Model file for the job. Use its own axes, mm. A direction names the side the tool comes from. Give positions to 0.01 mm unless a question says otherwise; leave off trailing zeros. Use CSV: the item, a comma, the result in double quotes.
Autodesk Inventor part; units mm, degrees
ref_plane "Work Plane1" through (16.3274, 9.3302, 5.6189) normal (-0.0349, 0, -0.9994) x (0, 1, 0)
ref_plane "YZ Plane" through (0, 0, 0) normal (1, 0, 0) x (0, 1, 0)
ref_plane "XZ Plane" through (0, 0, 0) normal (0, 1, 0) x (-1, 0, 0)
sketch "Sketch1" plane through (0, 0, 0) normal (0, 0, 1) x (1, 0, 0)
  line L0 (112.0815, -40.6698) -> (40.0716, -40.6698)
  line L1 (40.0716, -40.6698) -> (40.0716, 86.9433)
  line L2 (40.0716, 86.9433) -> (112.0815, 86.9433)
  line L3 (112.0815, 86.9433) -> (112.0815, -40.6698)
  line L4 (40.0716, -40.6698) -> (50.0716, -40.6698) construction
  point P0 (0, 0)
extrude "Extrusion1" add sketch "Sketch1" along normal blind 5.15
sketch "Sketch2" plane through (0, 0, 5.15) normal (0, 0, 1) x (1, 0, 0)
  point P0 (0, 0)
sketch "Sketch4" plane through (0, 0, 5.15) normal (0, 0, 1) x (1, 0, 0)
  circle A0 centre (102.6515, 97.6673) radius 2.8 construction
  circle A1 centre (53.4593, 78.9433) radius 2.8 construction
  circle A2 centre (55.5115, 50.5273) radius 2.8 construction
  circle A3 centre (102.6515, 50.5273) radius 2.8 construction
  line L0 (53.4593, 78.9433) -> (53.4593, 75.9433) construction
  line L1 (50.6593, 78.9433) -> (50.6593, 75.9433)
  line L2 (56.2593, 75.9433) -> (56.2593, 78.9433)
  arc A4 (56.2593, 78.9433) -> (50.6593, 78.9433) centre (53.4593, 78.9433) ccw
  arc A5 (50.6593, 75.9433) -> (56.2593, 75.9433) centre (53.4593, 75.9433) ccw
  line L3 (40.0716, 86.9433) -> (40.0716, -40.6698)
  line L4 (112.0815, 86.9433) -> (40.0716, 86.9433)
  circle A6 centre (53.4593, 77.3133) radius 5
  line L5 (53.4593, 77.3133) -> (53.4593, 77.5733) construction
  point P0 (0, 0)
  point P1 (53.4593, 77.4433)
  point P2 (40.0716, -42.6698)
  point P3 (53.4593, 77.4433)
  dimension "d7" = 3
  dimension "d27" = 5.6
  dimension "d29" = 8
extrude "Extrusion3" cut sketch "Sketch4" against normal through all contours A4 L2 A5 L1
pattern_linear "Rectangular Pattern1" count 2 spacing 47.14 along (1, 0, 0) count 2 spacing 47.14 along (0, -1, 0) of "Extrusion3"
sketch "Sketch9" plane through (0, 0, 5.15) normal (0, 0, 1) x (1, 0, 0)
  point P0 (55.0716, -3.0051)
  point P1 (44.0716, -3.0051)
  point P2 (44.0716, -19.0051)
  point P3 (44.0716, -35.0051)
  point P4 (44.0716, 36.9949)
hole "Hole1" at (55.0716, -3.0051, 5.15) at (44.0716, -3.0051, 5.15) at (44.0716, -19.0051, 5.15) at (44.0716, -35.0051, 5.15) at (44.0716, 36.9949, 5.15) direction (0, 0, -1) diameter 4.4 depth 5.15
sketch "Sketch12" plane through (0, 0, 5.15) normal (0, 0, 1) x (1, 0, 0)
  line L0 (40.0716, -40.6698) -> (112.0815, -40.6698)
  arc A0 (112.0815, 21.0326) -> (61.7828, -40.6698) centre (221.9091, -119.8494) ccw
  line L1 (112.0815, -40.6698) -> (112.0815, 86.9433)
  point P0 (0, 0)
extrude "Extrusion9" cut sketch "Sketch12" against normal through all
fillet "Fillet1" radius 8 2 edges at (61.7828, -40.6698, 2.575) (112.0815, 21.0326, 2.575)
ref_plane "Work Plane1" through (16.3274, 9.3302, 5.6189) normal (-0.0349, 0, -0.9994) x (0, 1, 0)
sketch "Sketch14" plane through (40.0716, -40.6698, 0) normal (-1, 0, 0) x (0, 0, 1)
  line L0 (0, 0) -> (0, 127.6131)
  line L1 (0, 0) -> (5.15, 0)
  line L2 (5.15, 127.6131) -> (5.15, 0)
  line L3 (0, 127.6131) -> (5.15, 127.6131)
  point P0 (0, 40.6698)
extrude "Extrusion11" add sketch "Sketch14" along normal blind 4
fillet "Fillet4" radius 4 1 edges at (36.0716, -40.6698, 2.575)
fillet "Fillet5" radius 6 2 edges at (36.0716, 86.9433, 2.575) (112.0815, 86.9433, 2.575)
sketch "Sketch15" plane through (0, 0, 0) normal (0, 0, -1) x (-1, 0, 0)
  circle A0 centre (-77.0293, 53.7433) radius 3.175 construction
  circle A1 centre (-77.0293, 53.7433) radius 3.175 construction
  circle A2 centre (-77.0293, 53.7433) radius 3.475 construction
  circle A3 centre (-77.0293, 53.7433) radius 3.475 construction
  circle A4 centre (-77.0293, 53.7433) radius 4.765
  point P0 (0, 0)
  dimension "d67" = 9.53
extrude "Extrusion12" cut sketch "Sketch15" against normal through all
sketch "Sketch16" plane through (0, 0, 5.15) normal (0, 0, 1) x (1, 0, 0)
  circle A0 centre (76.6012, 9.7443) radius 6.1
  point P0 (0, 0)
  dimension "d68" = 12.2
extrude "Extrusion13" cut sketch "Sketch16" against normal through all
sketch "Sketch17" plane through (0, 0, 0) normal (0, 0, -1) x (-1, 0, 0)
  circle A0 centre (-76.7219, 9.782) radius 12.5
  point P0 (0, 0)
  dimension "d71" = 25
extrude "Extrusion14" cut sketch "Sketch17" against normal blind 2.75
sketch "Sketch18" plane through (0, 0, 0) normal (0, 0, -1) x (-1, 0, 0)
  circle A0 centre (-92.5293, 69.2433) radius 1.25 construction
  circle A1 centre (-61.5293, 69.2433) radius 1.25 construction
  circle A2 centre (-92.5293, 38.2433) radius 1.25 construction
  circle A3 centre (-61.5293, 38.2433) radius 1.25 construction
  point P0 (0, 0)
hole "Hole2" at (92.5293, 69.2433, 0) at (61.5293, 69.2433, 0) at (61.5293, 38.2433, 0) at (92.5293, 38.2433, 0) direction (0, 0, 1) diameter 3.3 depth 6
chamfer "Chamfer1" distance 0.5 angle 45 28 edges at (81.7943, 53.7433, 0) (89.2219, 9.782, 0) (70.5012, 9.7443, 2.75) (100.5993, 26.0033, 0) (103.3993, 30.3033, 0) (100.5993, 34.6033, 0) (97.7993, 30.3033, 0) (61.5293, 36.5933, 0) (61.5293, 67.5933, 0) (92.5293, 36.5933, 0) (92.5293, 67.5933, 0) (53.4593, 26.0033, 0) (56.2593, 30.3033, 0) (53.4593, 34.6033, 0) (50.6593, 30.3033, 0) (44.0716, -32.8051, 0) (44.0716, -16.8051, 0) (44.0716, -0.8051, 0) (55.0716, -0.8051, 0) (44.0716, 39.1949, 0) (100.5993, 73.1433, 0) (103.3993, 77.4433, 0) (100.5993, 81.7433, 0) (97.7993, 77.4433, 0) (53.4593, 73.1433, 0) (56.2593, 77.4433, 0) (53.4593, 81.7433, 0) (50.6593, 77.4433, 0)
chamfer "Chamfer2" distance 0.5 angle 45 9 edges at (83.7732, -6.5873, 0) (61.0183, -39.5216, 0) (48.4802, -40.6698, 0) (36.0716, 22.1368, 0) (37.829, 85.186, 0) (74.0766, 86.9433, 0) (110.3242, 85.186, 0) (112.0815, 52.9152, 0) (111.3067, 21.4523, 0)
sketch "Sketch19" plane through (0, 0, 5.15) normal (0, 0, 1) x (1, 0, 0)
  circle A0 centre (44.0716, 62.6897) radius 2.2
  circle A1 centre (44.0716, 36.9949) radius 2.2 construction
  point P0 (0, 0)
  dimension "d87" = 4.4
extrude "Extrusion15" cut sketch "Sketch19" against normal through all
properties part number "XMotorMount" material "Aluminum 6061"
(1) Saw through at A-A, the plane x = 79. Count the separate pieces of the cut face and the enclosed holes in it, then the cut area to 3 significant figures.
Checked values:
separate pieces,"3"
enclosed holes,"0"
area,"373 mm^2"
(2) Wall check: probe 1 along Y at (x, z) = (44, 2.05); probe 2 along Y at (x, z) = (54.5, 0.3); probe 3 along X at (y, z) = (63, 2.5). Give the ranges that are in metal, low to high. Write a range as [from, to].
Checked values:
probe 1,"y = [-40.67, -37.2], [-32.81, -21.2], [-16.81, -5.2], [-0.81, 34.8], [39.19, 60.49], [64.89, 86.94]"
probe 2,"y = [-40.47, -5.34], [-0.67, 25.99], [34.62, 73.13], [81.76, 86.74]"
probe 3,"x = [36.07, 41.89], [46.25, 112.08]"
(3) 3-axis set-ups, long thin cutter, end or side, ignore diameter. For faces 1 (the face through (100.664, 25.862, 0.358)), 2 (the face through (84.09, -6.2, 2.86)), 3 (the face through (50.659, 30, 3)): which of +Z, -Z, +X, -X, +Y, -Y reach the whole face in a straight line?
Checked values:
face 1,"-Z"
face 2,"+Z, -Z, +X, -Y"
face 3,"+Z, -Z"
(4) Pull direction Y, two halves, no side cores. Call faces 4 (the face through (61.07, -39.49, 2.79)), 5 (the face through (66, 36, 0)), 6 (the face through (53.39, 34.74, 0.36)): released by +Y, released by -Y, zero draft, split by the parting line, or undercut.
Checked values:
face 4,"released by -Y"
face 5,"zero draft"
face 6,"undercut"
(5) Flat gauge pins, fed straight in: P1, Ø3.5, axis at x = 44.07, y = 36.99, coming from the -Z side; P2, Ø2, axis at x = 80.5, z = 2, coming from the -Y side. Where does each tip first touch, or does it go through?
Checked values:
P1,"passes through"
P2,"stops at y = -12.01"
